CAD build for the part. Positions are in the model's coordinates, mm. Round coordinates to 2 decimals unless told otherwise and drop trailing zeros. Write each loop counter-clockwise with the first axis right and the second up, starting at its lowest first coordinate (ties: lowest second). Pieces come first, ordered by that corner, then holes. Notation, with made-up numbers: M 31.25,77.5 L 71.25,77.5 A30 ccw 71.25,111.5 Z; hole C -13.75,71.25 d9. An arc over 180 degrees is marked long. Write each question's results on one line, items separated by ' | '. Start each with the question number.
```python
from build123d import *

# Parameters (mm, degrees)
SKETCH_1_R               = 15
SKETCH_1_R_2             = 13.5
EXTRUDE_1_DEPTH          = 299.33
CUT_EXTRUDE_1_DEPTH      = 301.080737302
CUT_EXTRUDE_1_DEPTH_BACK = 301.080737302
SKETCH_2_R               = 1.55
CUT_EXTRUDE_2_DEPTH      = 301.080737413
CUT_EXTRUDE_2_DEPTH_BACK = 301.080737413
SKETCH_3_R               = 2.1


with BuildPart() as part:
    # 草图1 → 凸台-拉伸1 (new body)
    with BuildSketch(Plane.XY):
        Circle(SKETCH_1_R)
        Circle(SKETCH_1_R_2, mode=Mode.SUBTRACT)
    extrude(amount=EXTRUDE_1_DEPTH)

    # 草图2 → 切除-拉伸1 (cut, two sides: drawn at the far end of the back side and taken through both)
    with BuildSketch(Plane(origin=(0, 0, 0), x_dir=(0, 0, -1), z_dir=(1, 0, 0)).offset(-CUT_EXTRUDE_1_DEPTH_BACK)):
        with Locations((-15.1, 0)):
            Circle(SKETCH_2_R)
        with Locations((-58.1, 0)):
            Circle(SKETCH_2_R)
    extrude(amount=CUT_EXTRUDE_1_DEPTH + CUT_EXTRUDE_1_DEPTH_BACK, mode=Mode.SUBTRACT)

    # 草图3 → 切除-拉伸2 (cut, two sides: drawn at the far end of the back side and taken through both)
    with BuildSketch(Plane(origin=(0, 0, 0), x_dir=(0, 0, -1), z_dir=(1, 0, 0)).offset(-CUT_EXTRUDE_2_DEPTH_BACK)):
        with Locations((-229.33, 0)):
            Circle(SKETCH_3_R)
    extrude(amount=CUT_EXTRUDE_2_DEPTH + CUT_EXTRUDE_2_DEPTH_BACK, mode=Mode.SUBTRACT)


solid = part.part
```
1) Wall check: line 1 along Z through (x, y) = (14.55, 0); line 2 along Y through (x, z) = (-1, 18). Give the ranges that are in metal, low to high. Write a range as from..to.
2) Drop flat-ended pins along their axis: pin 1 Ø3 at (x, z) = (-2, 163) entering from -Y; pin 2 Ø10 at (x, z) = (-9, 66) entering from +Y; pin 3 Ø1 at (y, z) = (-8, 260.5) entering from -X; pin 4 Ø1.9 at (y, z) = (0, 58.1) entering from -X. Give the stop position or say it passes through.
3) Saw through at A-A, the plane x = 0. Write the cut outline in (y, z), plus the area to 3 significant figures.
4) Saw through at B-B, the plane y = -8. Write the cut outline in (x, z).
5) Saw through at C-C, the plane z = 114. Write the cut outline in (x, y).
6) Pull direction X, two halves, no side cores. Call faces 1 (the face through (12.47, -5.17, 147.57)), 2 (the face through (-11.18, 7.85, 0)), 3 (the face through (14.307, 4.506, 147.57)): pulls with the +X half, pulls with the -X half, needs draft (parallel to the pull), parting line crosses it, or undercut.
Filled sheet:
1) line 1: z = 0..13.55, 16.65..56.55, 59.65..227.23, 231.43..299.33 | line 2: y = -14.97..-13.46, 13.46..14.97
2) pin 1: stops at y = -14.99 | pin 2: stops at y = 14.46 | pin 3: stops at x = -12.99 | pin 4: passes through
3) outline: M -15,0 L -13.5,0 L -13.5,299.33 L -15,299.33 Z; M 13.5,0 L 15,0 L 15,299.33 L 13.5,299.33 Z | area: 898 mm^2
4) outline: M -12.69,0 L -10.87,0 L -10.87,299.33 L -12.69,299.33 Z; M 10.87,0 L 12.69,0 L 12.69,299.33 L 10.87,299.33 Z
5) outline: C 0,0 d30; hole C 0,0 d27
6) face 1: undercut | face 2: needs draft | face 3: parting line crosses it
